```python
from build123d import *

# Parameters (mm, degrees)
SKETCH_W      = 92.1334
SKETCH_H      = 84.09
PAD_DEPTH     = 25.4
FILLET_R      = 3
SKETCH001_W   = 90.133333
SKETCH001_H   = 84.09
SKETCH001_W_2 = 92.133365
SKETCH001_H_2 = 82.09
SKETCH001_W_3 = 89.13332
SKETCH001_W_4 = 92.1334
PAD001_DEPTH  = 8


with BuildPart() as part:
    # Sketch → Pad (new body)
    with BuildSketch(Plane.XY):
        Polygon((-140.19998, 86.09), (-48.066647, 86.09), (-48.066647, 170.18), (-140.19998, 170.18), (-140.19998, 172.18), (139.20002, 172.18), (139.20002, 170.18), (48.0667, 170.18), (48.0667, 86.09), (139.20002, 86.09), (139.20002, 84.09), (48.066665, 84.09), (48.066665, 0), (46.066665, 0), (46.066665, 84.09), (-46.06665, 84.09), (-46.06665, 0), (-48.06665, 0), (-48.06665, 84.09), (-140.19998, 84.09), align=None)
        with Locations((0, 128.135)):
            Rectangle(SKETCH_W, SKETCH_H, mode=Mode.SUBTRACT)
    extrude(amount=PAD_DEPTH)

    # Fillet
    fillet_edges = [part.edges().sort_by_distance(p)[0] for p in [
        (-47.06665, 0, 25.4),
        (47.066665, 0, 25.4),
        (139.20002, 171.18, 25.4),
        (139.20002, 85.09, 25.4),
        (-140.19998, 85.09, 25.4),
        (-140.19998, 171.18, 25.4),
    ]]
    fillet(fillet_edges, radius=FILLET_R)

    # Sketch001 → Pad001 (join)
    with BuildSketch(Plane.XY):
        Polygon((139.20002, 86.09), (139.20002, 84.09), (48.066665, 0), (46.066665, 0), (-46.06665, 0), (-48.06665, 0), (-140.19998, 84.09), (-140.19998, 86.09), (-140.19998, 170.18), (-140.19998, 172.18), (139.20002, 172.18), (139.20002, 170.18), align=None)
        with Locations((-93.133313, 128.135)):
            Rectangle(SKETCH001_W, SKETCH001_H, mode=Mode.SUBTRACT)
        Polygon((137.20002, 84.09), (48.066665, 84.09), (48.066665, 2), align=None, mode=Mode.SUBTRACT)
        with Locations((-1.7e-05, 43.045)):
            Rectangle(SKETCH001_W_2, SKETCH001_H_2, mode=Mode.SUBTRACT)
        Polygon((-48.0667, 2), (-48.0667, 84.09), (-138.19998, 84.09), align=None, mode=Mode.SUBTRACT)
        with Locations((92.63336, 128.135)):
            Rectangle(SKETCH001_W_3, SKETCH001_H, mode=Mode.SUBTRACT)
        with Locations((0, 128.135)):
            Rectangle(SKETCH001_W_4, SKETCH001_H, mode=Mode.SUBTRACT)
    extrude(amount=PAD001_DEPTH)


solid = part.part
```
Work out the finished part from the listing and answer in its coordinate system (mm). A direction names the side the tool comes from. Give positions to 0.01 mm unless a question says otherwise; leave off trailing zeros. Loops run counter-clockwise (first coordinate to the right, second up) from the corner with the lowest first, then second, coordinate; pieces in that order, holes last. Notation, with made-up numbers: (-29.5, 59) - (-10.5, 59) arc R23 ccw to (-10.5, 86) - close; hole circle Ø11 at (6.25, 5.25). An arc over 180 degrees is marked (long way). Use CSV: the item, a comma, the result in double quotes. Start each with the question number.
(1) Find section A-A, the plane y = 116. Determine the outline of the cut face in (x, z), plus the area to 3 significant figures.
(2) Find section B-B, the plane z = 19. Determine the outline of the cut face in (x, y).
(3) Find section D-D, the plane x = -79.5. Determine the outline of the cut face in (y, z).
(4) Each of these flat-tipped pins is pushed along its axis until it touches: pin 1 (7.5 mm diameter, centred on x = 87, z = 10.5, fed in from -Y); pin 2 (12.5 mm diameter, centred on x = -85, z = 18, fed in from -Y); pin 3 (10 mm diameter, centred on y = 41.5, z = 19, fed in from +X). Where does it stop, or does it pass through?
(5) Find section C-C, the plane x = 55. Determine the outline of the cut face in (y, z), plus the area to 3 significant figures.
(6) Find the intervals of material crossed by L1, parallel to Y at x = 41, z = 3.5; L2, parallel to X at y = 143.5, z = 3; L3, parallel to Y at x = 59, z = 23, in increasing order.
(7) A tool of negligible diameter and unlimited length cuts with its end or side. For faces 1 (the face through (-93.49, 41.46, 3.94)), 2 (the face through (-93.764, 43.62, 3.944)), 3 (the face through (-93.9, 42.2, 8)), from which of +Z, -Z, +X, -X, +Y, -Y can it reach the whole face along a straight path? Write none if from no direction.
(8) Determine the mould class of faces 4 (the face through (139.2, 128, 6)), 5 (the face through (93, 86.09, 13)), 6 (the face through (94.27, 42.63, 3.94)) for opening direction Y: released by +Y, released by -Y, zero draft, split by the parting line, or undercut.
Results found:
1,outline,"(-140.2, 0) - (-138.2, 0) - (-138.2, 8) - (-140.2, 8) - close; (-48.07, 0) - (-46.07, 0) - (-46.07, 25.4) - (-48.07, 25.4) - close; (46.07, 0) - (48.07, 0) - (48.07, 25.4) - (46.07, 25.4) - close; (137.2, 0) - (139.2, 0) - (139.2, 8) - (137.2, 8) - close"
1,area,"134 mm^2"
2,outline,"(-140.2, 84.09) - (-48.07, 84.09) - (-48.07, 0) - (-46.07, 0) - (-46.07, 84.09) - (46.07, 84.09) - (46.07, 0) - (48.07, 0) - (48.07, 84.09) - (139.2, 84.09) - (139.2, 86.09) - (48.07, 86.09) - (48.07, 170.18) - (139.2, 170.18) - (139.2, 172.18) - (-140.2, 172.18) - (-140.2, 170.18) - (-48.07, 170.18) - (-48.07, 86.09) - (-140.2, 86.09) - close; hole (-46.07, 86.09) - (46.07, 86.09) - (46.07, 170.18) - (-46.07, 170.18) - close"
3,outline,"(28.69, 0) - (30.63, 0) - (30.63, 8) - (28.69, 8) - close; (84.09, 0) - (86.09, 0) - (86.09, 25.4) - (84.09, 25.4) - close; (170.18, 0) - (172.18, 0) - (172.18, 25.4) - (170.18, 25.4) - close"
4,pin 1,"y = 33.35"
4,pin 2,"y = 84.09"
4,pin 3,"x = 48.07"
5,outline,"(6.4, 0) - (8.39, 0) - (8.39, 8) - (6.4, 8) - close; (84.09, 0) - (86.09, 0) - (86.09, 25.4) - (84.09, 25.4) - close; (170.18, 0) - (172.18, 0) - (172.18, 25.4) - (170.18, 25.4) - close"
5,area,"118 mm^2"
6,L1,"0 to 2, 84.09 to 86.09, 170.18 to 172.18"
6,L2,"-140.2 to -138.2, -48.07 to -46.07, 46.07 to 48.07, 137.2 to 139.2"
6,L3,"84.09 to 86.09, 170.18 to 172.18"
7,face 1,"+Z, -Z, -X, -Y"
7,face 2,"+Z, -Z"
7,face 3,"+Z, -X, -Y"
8,face 4,"zero draft"
8,face 5,"undercut"
8,face 6,"released by -Y"
